Answer from the drawing. Dimensions are ordinates in mm from the lowest x, y and z of the part. A direction names the side the tool comes from. Coordinates: 2 decimals unless noted, no trailing zeros. Write each loop counter-clockwise with the first axis right and the second up, starting at its lowest first coordinate (ties: lowest second). Pieces come first, ordered by that corner, then holes.
(1) Which of the six approach directions +Z, -Z, +X, -X, +Y, -Y give full straight-line access (tool end or side, diameter ignored) to the marked faces 1 and 2?
(2) Given P1, Ø2, axis at y = 8.5, z = 22.5, coming from the +X side; P2, Ø6, axis at x = 64.5, z = 30, coming from the +Y side, each flat-ended and moving along its own axis, determine where each tip first touches the part or whether it passes through.
(3) The part is cut by section C-C on x = 80.5. Determine the outline of the cut face in (y, z), plus the area to 3 significant figures.
(4) Straight lines are drawn through the part: line 1 (X direction, y = 8.75, z = 5.5); line 2 (Y direction, x = 110, z = 52). For each, find the intervals that lie inside material, in ascending order.
(5) The part is cut by section A-A on z = 22. Determine the outline of the cut face in (x, y).
(6) The part is cut by section B-B on y = 8.5. Determine the outline of the cut face in (x, z).
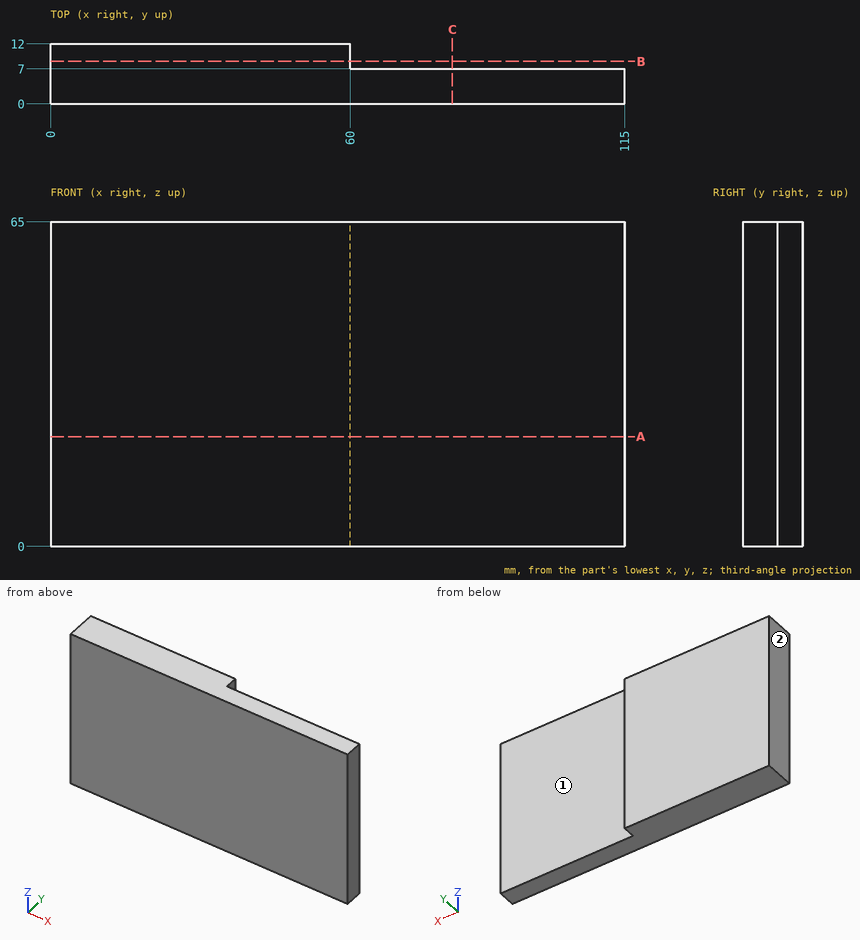
Model answer:
1. face 1: +Z, -Z, +X, +Y
1. face 2: +Z, -Z, -X, +Y, -Y
2. P1: stops at x = 60
2. P2: stops at y = 7
3. outline: (0, 0) - (7, 0) - (7, 65) - (0, 65) - close
3. area: 455 mm2
4. line 1: x = 0 to 60
4. line 2: y = 0 to 7
5. outline: (0, 0) - (115, 0) - (115, 7) - (60, 7) - (60, 12) - (0, 12) - close
6. outline: (0, 0) - (60, 0) - (60, 65) - (0, 65) - close
